from build123d import *

# Parameters (mm, degrees)
SKETCH1_R           = 1.65
BOSS_EXTRUDE1_DEPTH = 3


with BuildPart() as part:
    # Sketch1 → Boss-Extrude1 (new body)
    with BuildSketch(Plane.XY):
        with BuildLine():
            ThreePointArc((-20.755142163, -16.478801884), (-21.932583818, -17.847935828), (-22.52081897, -19.555236625))
            ThreePointArc((-22.52081897, -19.555236625), (-22.269390429, -19.802297923), (-22.01159712, -20.042710497))
            ThreePointArc((-22.01159712, -20.042710497), (-20.331579752, -19.3805638), (-19.015108204, -18.144522024))
            ThreePointArc((-19.015108204, -18.144522024), (-18.373585411, -18.588879433), (-17.699741584, -18.98250298))
            ThreePointArc((-17.699741584, -18.98250298), (-18.263610953, -20.698005222), (-18.153713641, -22.500453331))
            ThreePointArc((-18.153713641, -22.500453331), (-17.826877693, -22.63249067), (-17.496705822, -22.755949699))
            ThreePointArc((-17.496705822, -22.755949699), (-16.197964732, -21.501291105), (-15.454716323, -19.855545556))
            ThreePointArc((-15.454716323, -19.855545556), (-14.691978327, -20.020578127), (-13.918794597, -20.126369997))
            ThreePointArc((-13.918794597, -20.126369997), (-13.78324768, -21.927070872), (-12.991948773, -23.550259908))
            ThreePointArc((-12.991948773, -23.550259908), (-12.639463228, -23.547171801), (-12.287178469, -23.534881765))
            ThreePointArc((-12.287178469, -23.534881765), (-11.567435216, -21.878721672), (-11.510562778, -20.073822192))
            ThreePointArc((-11.510562778, -20.073822192), (-10.742729525, -19.934405211), (-9.987916106, -19.736259551))
            ThreePointArc((-9.987916106, -19.736259551), (-9.173588692, -21.348018674), (-7.821356276, -22.544832821))
            ThreePointArc((-7.821356276, -22.544832821), (-7.496883863, -22.407089403), (-7.176118378, -22.260921351))
            ThreePointArc((-7.176118378, -22.260921351), (-7.144947346, -20.455395119), (-7.783109193, -18.766121291))
            ThreePointArc((-7.783109193, -18.766121291), (-7.127076334, -18.343479732), (-6.505546727, -17.871562422))
            ThreePointArc((-6.505546727, -17.871562422), (-5.136412783, -19.049004077), (-3.429111986, -19.637239229))
            ThreePointArc((-3.429111986, -19.637239229), (-3.182050688, -19.385810688), (-2.941638114, -19.128017379))
            ThreePointArc((-2.941638114, -19.128017379), (-3.603784812, -17.448000011), (-4.839826587, -16.131528463))
            ThreePointArc((-4.839826587, -16.131528463), (-4.395469179, -15.49000567), (-4.001845631, -14.816161843))
            ThreePointArc((-4.001845631, -14.816161843), (-2.286343389, -15.380031212), (-0.48389528, -15.2701339))
            ThreePointArc((-0.48389528, -15.2701339), (-0.351857941, -14.943297952), (-0.228398912, -14.613126081))
            ThreePointArc((-0.228398912, -14.613126081), (-1.483057507, -13.314384991), (-3.128803055, -12.571136582))
            ThreePointArc((-3.128803055, -12.571136582), (-2.963770485, -11.808398586), (-2.857978614, -11.035214856))
            ThreePointArc((-2.857978614, -11.035214856), (-1.05727774, -10.899667939), (0.565911297, -10.108369033))
            ThreePointArc((0.565911297, -10.108369033), (0.56282319, -9.755883487), (0.550533154, -9.403598729))
            ThreePointArc((0.550533154, -9.403598729), (-1.105626939, -8.683855475), (-2.910526419, -8.626983037))
            ThreePointArc((-2.910526419, -8.626983037), (-3.0499434, -7.859149784), (-3.24808906, -7.104336365))
            ThreePointArc((-3.24808906, -7.104336365), (-1.636329937, -6.290008951), (-0.43951579, -4.937776535))
            ThreePointArc((-0.43951579, -4.937776535), (-0.577259208, -4.613304122), (-0.723427261, -4.292538637))
            ThreePointArc((-0.723427261, -4.292538637), (-2.528953492, -4.261367605), (-4.21822732, -4.899529452))
            ThreePointArc((-4.21822732, -4.899529452), (-4.64086888, -4.243496594), (-5.112786189, -3.621966986))
            ThreePointArc((-5.112786189, -3.621966986), (-3.935344534, -2.252833042), (-3.347109382, -0.545532245))
            ThreePointArc((-3.347109382, -0.545532245), (-3.598537923, -0.298470947), (-3.856331232, -0.058058373))
            ThreePointArc((-3.856331232, -0.058058373), (-5.5363486, -0.720205071), (-6.852820148, -1.956246846))
            ThreePointArc((-6.852820148, -1.956246846), (-7.494342941, -1.511889438), (-8.168186768, -1.11826589))
            ThreePointArc((-8.168186768, -1.11826589), (-7.604317399, 0.597236351), (-7.714214711, 2.399684461))
            ThreePointArc((-7.714214711, 2.399684461), (-8.041050659, 2.5317218), (-8.37122253, 2.655180829))
            ThreePointArc((-8.37122253, 2.655180829), (-9.66996362, 1.400522234), (-10.413212029, -0.245223314))
            ThreePointArc((-10.413212029, -0.245223314), (-11.175950025, -0.080190744), (-11.949133755, 0.025601127))
            ThreePointArc((-11.949133755, 0.025601127), (-12.084680673, 1.826302001), (-12.875979579, 3.449491038))
            ThreePointArc((-12.875979579, 3.449491038), (-13.228465124, 3.44640293), (-13.580749883, 3.434112895))
            ThreePointArc((-13.580749883, 3.434112895), (-14.300493136, 1.777952801), (-14.357365574, -0.026946679))
            ThreePointArc((-14.357365574, -0.026946679), (-15.125198828, -0.166363659), (-15.880012246, -0.364509319))
            ThreePointArc((-15.880012246, -0.364509319), (-16.69433966, 1.247249804), (-18.046572076, 2.444063951))
            ThreePointArc((-18.046572076, 2.444063951), (-18.371044489, 2.306320533), (-18.691809974, 2.16015248))
            ThreePointArc((-18.691809974, 2.16015248), (-18.722981006, 0.354626248), (-18.084819159, -1.334647579))
            ThreePointArc((-18.084819159, -1.334647579), (-18.740852018, -1.757289139), (-19.362381625, -2.229206448))
            ThreePointArc((-19.362381625, -2.229206448), (-20.731515569, -1.051764793), (-22.438816366, -0.463529641))
            ThreePointArc((-22.438816366, -0.463529641), (-22.685877664, -0.714958182), (-22.926290238, -0.972751491))
            ThreePointArc((-22.926290238, -0.972751491), (-22.264143541, -2.652768859), (-21.028101765, -3.969240407))
            ThreePointArc((-21.028101765, -3.969240407), (-21.69320555, -4.973863328), (-22.234253204, -6.050384435))
            Line((-22.234253204, -6.050384435), (-52.933964176, -6.050384435))
            ThreePointArc((-52.933964176, -6.050384435), (-56.933964176, -10.050384435), (-52.933964176, -14.050384435))
            Line((-52.933964176, -14.050384435), (-22.234253204, -14.050384435))
            ThreePointArc((-22.234253204, -14.050384435), (-21.580377364, -15.316779311), (-20.755142163, -16.478801884))
        make_face()
        with Locations((-12.933964176, -10.050384435)):
            Circle(SKETCH1_R, mode=Mode.SUBTRACT)
        with Locations((-52.933964176, -10.050384435)):
            Circle(SKETCH1_R, mode=Mode.SUBTRACT)
    extrude(amount=BOSS_EXTRUDE1_DEPTH)


solid = part.part
Could you check a few things on this model? Use its own coordinates, in mm. A direction names the side the tool comes from. Give positions to 0.01 mm unless a question says otherwise; leave off trailing zeros. Order: outer loops, then holes, each group sorted by start corner. A loop starts at its lowest first (then second) coordinate and runs counter-clockwise, first axis right, second up. Notation, with made-up numbers: (-35, -6) -> (-18, -6) arc R21 cw to (-18, 27) -> close; hole circle Ø1 at (85.25, 73). An arc over 180 degrees is marked (long way). Answer in a Markdown table with one row per item. Add a question column.
Item 1: Please list where these lines run through material, in increasing order: probe 1 along X at (y, z) = (-1.5, 1.2); probe 2 along X at (y, z) = (0.25, 1.45); probe 3 along Y at (x, z) = (-23.5, 1.2).
Item 2: Imagine slicing it at B-B (z = 0.65). Count the separate pieces of the cut face and the enclosed holes in it, and give its area (3 significant figures).
Item 3: Imagine slicing it at A-A (x = -39). List the corners of the cut face in (y, z) for me.
Item 4: For faces 4 (the cylindrical face through (-9.189, -21.328, 1.479)), 5 (the cylindrical face through (-21.685, -4.959, 1.479)), 6 (the cylindrical face through (-7.136, -18.35, 1.479)), which set-ups out of +Z, -Z, +X, -X, +Y, -Y let a thin tool reach every point of the face, with its end or its side?
Item 5: We'd pull the mould along Y, two halves only. Please class faces 1 (the cylindrical face through (-20.35, -19.39, 1.48)), 2 (the cylindrical face through (-11.573, -21.904, 1.479)), 3 (the cylindrical face through (-9.655, 1.421, 1.479)): pulls with the +Y half, pulls with the -Y half, needs draft (parallel to the pull), parting line crosses it, or undercut.
Item 6: I'm going to push flat-ended pins straight in: P1, Ø1.5, axis at x = -35, y = -7.5, coming from the -Z side; P2, Ø1.5, axis at x = -41, z = 1, coming from the -Y side; P3, Ø1.5, axis at y = -19, z = 0.5, coming from the +X side. Where does each tip first touch, or does it pass through?
Result:
| question | item | result |
|---|---|---|
| 1 | probe 1 | -22.8 to -20.08, -18.35 to -7.51, -6.48 to -3.59 |
| 1 | probe 2 | -18.7 to -16.1, -14.39 to -11.93, -10.27 to -7.66 |
| 1 | probe 3 | -14.05 to -6.05 |
| 2 | separate pieces | 1 |
| 2 | enclosed holes | 2 |
| 2 | area | 660 mm2 |
| 3 | outline | (-14.05, 0) -> (-6.05, 0) -> (-6.05, 3) -> (-14.05, 3) -> close |
| 4 | face 4 | +Z, -Z, -Y |
| 4 | face 5 | +Z, -Z, -X |
| 4 | face 6 | +Z, -Z |
| 5 | face 1 | pulls with the -Y half |
| 5 | face 2 | undercut |
| 5 | face 3 | pulls with the +Y half |
| 6 | P1 | z = 0 |
| 6 | P2 | y = -14.05 |
| 6 | P3 | x = -2.94 |
